Autodesk Inventor part; units mm, degrees
ref_plane "YZ Plane" through (0, 0, 0) normal (1, 0, 0) x (0, 1, 0)
ref_plane "XZ Plane" through (0, 0, 0) normal (0, 1, 0) x (-1, 0, 0)
ref_plane "XY Plane" through (0, 0, 0) normal (0, 0, 1) x (1, 0, 0)
sketch "Sketch1" plane through (0, 0, 0) normal (0, 0, 1) x (1, 0, 0)
  line L0 (262.89, 253.3796) -> (525.78, 101.6)
  line L1 (525.78, 101.6) -> (525.78, -201.9592) construction
  line L2 (525.78, -201.9592) -> (262.89, -353.7388) construction
  line L3 (262.89, -353.7388) -> (0, -201.9592) construction
  line L4 (0, -201.9592) -> (0, 101.6) construction
  line L5 (0, 101.6) -> (262.89, 253.3796)
  line L6 (0, 101.6) -> (0, 0)
  line L7 (0, 0) -> (525.78, 0)
  line L8 (525.78, 0) -> (525.78, 101.6)
  point P0 (262.89, -50.1796)
  dimension "d0" = 525.78
  dimension "d1" = 101.6
extrude "Extrusion1" add sketch "Sketch1" along normal blind 25.4
sketch "Sketch2" plane through (0, 0, 25.4) normal (0, 0, 1) x (1, 0, 0)
  circle A0 centre (262.89, 121.3796) radius 60
  line L0 (0, 0) -> (525.78, 0)
  point P0 (262.89, 0)
  dimension "d4" = 121.3796
  dimension "d5" = 120
extrude "Extrusion2" cut sketch "Sketch2" against normal through all
sketch "Sketch3" plane through (0, 0, 25.4) normal (0, 0, 1) x (1, 0, 0)
  circle A0 centre (262.89, 121.3796) radius 60
  line L0 (0, 101.6) -> (0, 0)
  line L1 (0, 0) -> (525.78, 0)
  line L2 (525.78, 0) -> (525.78, 101.6)
  line L3 (525.78, 101.6) -> (262.89, 253.3796)
  line L4 (262.89, 253.3796) -> (0, 101.6)
  line L5 (25.4, 86.9353) -> (25.4, 25.4)
  line L6 (25.4, 25.4) -> (500.38, 25.4)
  line L7 (500.38, 25.4) -> (500.38, 86.9353)
  line L8 (500.38, 86.9353) -> (262.89, 224.0502)
  line L9 (262.89, 224.0502) -> (25.4, 86.9353)
  dimension "d8" = 25.4
extrude "Extrusion3" cut sketch "Sketch3" against normal through all contours L4 L3 L2 L1 L0
sketch "Sketch4" plane through (0, 0, 25.4) normal (0, 0, 1) x (1, 0, 0)
  line L0 (134.346, 149.8353) -> (159.746, 105.8412)
  line L1 (159.746, 105.8412) -> (115.7519, 80.4412)
  line L2 (115.7519, 80.4412) -> (90.3519, 124.4353)
  line L3 (90.3519, 124.4353) -> (134.346, 149.8353)
  line L4 (134.346, 149.8353) -> (115.7519, 80.4412) construction
  line L5 (159.746, 105.8412) -> (90.3519, 124.4353) construction
  line L6 (262.89, 224.0502) -> (25.4, 86.9353)
  line L7 (500.38, 86.9353) -> (262.89, 224.0502)
  line L8 (262.89, 224.0502) -> (262.89, 25.4)
  line L9 (25.4, 25.4) -> (500.38, 25.4)
  line L10 (391.434, 149.8353) -> (366.034, 105.8412)
  line L11 (366.034, 105.8412) -> (410.0281, 80.4412)
  line L12 (410.0281, 80.4412) -> (435.4281, 124.4353)
  line L13 (435.4281, 124.4353) -> (391.434, 149.8353)
  line L14 (391.434, 149.8353) -> (410.0281, 80.4412) construction
  line L15 (366.034, 105.8412) -> (435.4281, 124.4353) construction
  point P0 (0, 0)
  point P1 (125.049, 115.1383)
  point P2 (400.731, 115.1383)
  point P3 (381.635, 155.4928)
  dimension "d11" = 50.8
  dimension "d12" = 50.8
  dimension "d15" = 75
extrude "Extrusion4" cut sketch "Sketch4" against normal through all
sketch "Sketch5" plane through (0, 0, 0) normal (0, 0, -1) x (-1, 0, 0)
  line L0 (-25.4, 86.9353) -> (-25.4, 25.4)
  line L1 (-25.4, 43.4677) -> (-12.7, 43.4677)
  line L2 (-12.7, 43.4677) -> (-12.7, 68.8677)
  line L3 (-12.7, 68.8677) -> (-25.4, 68.8677)
  line L4 (-25.4, 68.8677) -> (-25.4, 43.4677)
  line L5 (-25.4, 25.4) -> (-500.38, 25.4)
  line L6 (-94.99, 25.4) -> (-120.39, 25.4)
  line L7 (-120.39, 25.4) -> (-120.39, 12.7)
  line L8 (-120.39, 12.7) -> (-94.99, 12.7)
  line L9 (-94.99, 12.7) -> (-94.99, 25.4)
  line L10 (-405.39, 25.4) -> (-430.79, 25.4)
  line L11 (-430.79, 25.4) -> (-430.79, 12.7)
  line L12 (-430.79, 12.7) -> (-405.39, 12.7)
  line L13 (-405.39, 12.7) -> (-405.39, 25.4)
  line L14 (-500.38, 25.4) -> (-500.38, 86.9353)
  line L15 (-500.38, 43.4677) -> (-513.08, 43.4677)
  line L16 (-513.08, 43.4677) -> (-513.08, 68.8677)
  line L17 (-513.08, 68.8677) -> (-500.38, 68.8677)
  line L18 (-500.38, 68.8677) -> (-500.38, 43.4677)
  line L19 (-262.89, 224.0502) -> (-134.346, 149.8353)
  line L20 (-198.618, 186.9428) -> (-220.615, 199.6428)
  line L21 (-220.615, 199.6428) -> (-214.265, 210.6413)
  line L22 (-214.265, 210.6413) -> (-192.268, 197.9413)
  line L23 (-192.268, 197.9413) -> (-198.618, 186.9428)
  line L24 (-391.434, 149.8353) -> (-262.89, 224.0502)
  line L25 (-305.165, 199.6428) -> (-327.162, 186.9428)
  line L26 (-327.162, 186.9428) -> (-333.512, 197.9413)
  line L27 (-333.512, 197.9413) -> (-311.515, 210.6413)
  line L28 (-311.515, 210.6413) -> (-305.165, 199.6428)
  line L29 (-262.89, 224.0502) -> (-391.434, 149.8353)
  line L30 (-120.39, 19.05) -> (-405.39, 19.05) construction
  line L31 (-250.19, 25.4) -> (-275.59, 25.4)
  line L32 (-275.59, 25.4) -> (-275.59, 12.7)
  line L33 (-275.59, 12.7) -> (-250.19, 12.7)
  line L34 (-250.19, 12.7) -> (-250.19, 25.4)
  line L35 (-500.38, 25.4) -> (-25.4, 25.4)
  line L36 (-305.165, 199.6428) -> (-311.515, 210.6413)
  line L37 (-311.515, 210.6413) -> (-333.512, 197.9413)
  line L38 (-333.512, 197.9413) -> (-327.162, 186.9428)
  line L39 (-327.162, 186.9428) -> (-305.165, 199.6428)
  point P0 (0, 0)
  point P1 (-25.4, 56.1677)
  point P2 (-262.89, 25.4)
  point P3 (-262.89, 19.05)
  point P4 (-262.89, 25.4)
  dimension "d16" = 12.7
  dimension "d17" = 12.7
  dimension "d18" = 12.7
  dimension "d19" = 12.7
  dimension "d20" = 12.7
  dimension "d21" = 12.7
  dimension "d22" = 25.4
  dimension "d23" = 25.4
  dimension "d24" = 25.4
  dimension "d25" = 25.4
  dimension "d26" = 25.4
  dimension "d27" = 25.4
  dimension "d28" = 285
  dimension "d29" = 25.4
  dimension "d30" = 12.7
extrude "Extrusion5" add sketch "Sketch5" against normal blind 25.4
sketch "Sketch6" plane through (0, 0, 0) normal (0, 0, -1) x (-1, 0, 0)
  line L0 (-275.59, 25.4) -> (-405.39, 25.4)
  line L1 (-324.58, 25.4) -> (-375.38, 25.4)
  line L2 (-375.38, 25.4) -> (-375.38, 76.2)
  line L3 (-375.38, 76.2) -> (-324.58, 76.2)
  line L4 (-324.58, 76.2) -> (-324.58, 25.4)
  line L5 (-500.38, 43.4677) -> (-500.38, 25.4)
  point P0 (0, 0)
  dimension "d33" = 50.8
  dimension "d34" = 50.8
  dimension "d35" = 125
extrude "Extrusion6" cut sketch "Sketch6" against normal through all
sketch "Sketch8" plane through (500.38, 86.9353, 25.4) normal (0.5, 0.866, 0) x (0.866, -0.5, 0)
  circle A0 centre (-248.8298, 12.7) radius 2
  circle A1 centre (-25.4, 12.7) radius 2
  line L0 (0, 0) -> (0, 25.4)
  line L1 (-274.2298, 0) -> (-274.2298, 25.4)
  point P0 (-389.8741, 25.4)
  point P1 (0, 12.7)
  dimension "d44" = 4
  dimension "d45" = 4
  dimension "d46" = 25.4
  dimension "d47" = 25.4
extrude "Extrusion8" cut sketch "Sketch8" against normal blind 38.1
sketch "Sketch9" plane through (262.89, 224.0502, 25.4) normal (-0.5, 0.866, 0) x (0.866, 0.5, 0)
  line L0 (0, 0) -> (0, 25.4)
  line L1 (-274.2298, 0) -> (-274.2298, 25.4)
  circle A0 centre (-25.4, 12.7) radius 2
  circle A1 centre (-248.8298, 12.7) radius 2
  point P0 (-339.6945, 25.4)
  point P1 (-274.2298, 12.7)
  dimension "d50" = 4
  dimension "d51" = 4
  dimension "d52" = 25.4
  dimension "d53" = 25.4
extrude "Extrusion9" cut sketch "Sketch9" against normal blind 38.1
sketch "Sketch10" plane through (500.38, 25.4, 25.4) normal (1, 0, 0) x (0, 0, -1)
  line L0 (0, 0) -> (25.4, 0)
  line L1 (0, 61.5353) -> (25.4, 61.5353)
  circle A0 centre (12.7, 8) radius 2
  circle A1 centre (12.7, 53.5353) radius 2
  point P0 (25.4, -25.4)
  point P1 (12.7, 0)
  point P2 (12.7, 61.5353)
  dimension "d56" = 4
  dimension "d57" = 4
  dimension "d58" = 8
  dimension "d59" = 8
extrude "Extrusion10" cut sketch "Sketch10" against normal blind 38.1
sketch "Sketch11" plane through (25.4, 86.9353, 0) normal (-1, 0, 0) x (0, 0, 1)
  circle A0 centre (12.7, -8) radius 2
  circle A1 centre (12.7, -53.5353) radius 2
  point P0 (0, -86.9353)
extrude "Extrusion11" cut sketch "Sketch11" against normal blind 38.1
sketch "Sketch12" plane through (120.39, 25.4, 25.4) normal (0, -1, 0) x (1, 0, 0)
  circle A0 centre (-60.195, -12.7) radius 2
  circle A1 centre (64.9, -12.7) radius 2
  circle A2 centre (345.195, -12.7) radius 2
  line L0 (310.4, 0) -> (379.99, 0)
  line L1 (0, 0) -> (129.8, 0)
  line L2 (-94.99, 0) -> (-25.4, 0)
  line L3 (379.99, 0) -> (379.99, -25.4)
  point P0 (-120.39, -25.4)
  point P1 (345.195, 0)
  point P2 (64.9, 0)
  point P3 (-60.195, 0)
  point P4 (379.99, -12.7)
  dimension "d64" = 4
  dimension "d65" = 4
  dimension "d66" = 4
extrude "Extrusion12" cut sketch "Sketch12" against normal blind 38.1
properties part number "HB04" material "Polyethylene, High Density"
Here's how the part is built. I have some questions about the finished solid (model axes, mm). A direction names the side the tool comes from. Round coordinates to 2 decimals unless told otherwise and drop trailing zeros. Order: outer loops, then holes, each group sorted by start corner. A loop starts at its lowest first (then second) coordinate and runs counter-clockwise, first axis right, second up. Notation, with made-up numbers: (59, 27.5) -> (92, 27.5) arc R35 ccw to (92, 60.5) -> close; hole circle Ø8 at (-23.5, 55). An arc over 180 degrees is marked (long way). Return JSON: item names as keys, results as strings.
Q1. If we section it at D-D on x = 418: List the corners of the cut face in (y, z) for me, plus the area to 3 significant figures.
Filled sheet:
{"outline": "(12.7, 0) -> (94.25, 0) -> (94.25, 25.4) -> (12.7, 25.4) -> close", "area": "2,070 mm^2"}
Q2. If we section it at B-B on x = 299: List the corners of the cut face in (y, z) for me, plus the area to 3 significant figures.
Filled sheet:
{"outline": "(25.4, 0) -> (73.46, 0) -> (73.46, 25.4) -> (25.4, 25.4) -> close; (169.3, 0) -> (203.2, 0) -> (203.2, 25.4) -> (169.3, 25.4) -> close", "area": "2,080 mm^2"}
Q3. Which directions (+Z, -Z, +X, -X, +Y, -Y) give clear straight access to the entire face, cutting with the end or side of a thin tool? Please do faces 4 (the flat face through (500.38, 76, 13)), 5 (the flat face through (103.23, 102.13, 12.88)), 6 (the flat face through (146.868, 128.146, 12.878)).
Filled sheet:
{"face 4": "+Z, -Z, +X, +Y", "face 5": "+Z, -Z, +Y", "face 6": "+Z, -Z"}
Q4. I need wall thicknesses on line 1 along Z through (x, y) = (49, 33); line 2 along Y through (x, z) = (487, 12.7); line 3 along X through (y, z) = (87.5, 3.5). Which ranges of each line are inside material? Lowest first, please. Write a range as from..to.
Filled sheet:
{"line 1": "z = 0..10.74, 14.66..25.4", "line 2": "y = 25.4..31.4, 35.4..76.94, 80.94..94.66", "line 3": "x = 26.38..111.68, 127.98..213.37, 312.41..397.8, 414.1..499.4"}
Q5. If we mould it in two halves opening along X, with no side actions, what happens to faces 1 (the flat face through (19, 68.868, 13)), 2 (the flat face through (203.42, 204.38, 12.52)), 3 (the flat face through (324.58, 51, 13))? For each: released by +X, released by -X, zero draft, split by the parting line, or undercut.
Filled sheet:
{"face 1": "zero draft", "face 2": "released by -X", "face 3": "undercut"}
Q6. For pin 1 Ø3.5 at (y, z) = (78.94, 12.7) entering from +X; pin 2 Ø3 at (y, z) = (34, 12) entering from +X; pin 3 Ø10 at (y, z) = (18, 8.5) entering from +X, each with a flat end and sliding along its axis, tell me the tip position at first contact or that it passes through.
Filled sheet:
{"pin 1": "stops at x = 462.28", "pin 2": "stops at x = 500.38", "pin 3": "stops at x = 430.79"}
Q7. If we section it at A-A on y = 175.5: List the corners of the cut face in (x, z) for me.
Filled sheet:
{"outline": "(178.8, 0) -> (236.99, 0) -> (236.99, 25.4) -> (178.8, 25.4) -> close; (288.79, 0) -> (346.98, 0) -> (346.98, 25.4) -> (288.79, 25.4) -> close"}
Q8. If we section it at C-C on y = 94: Give the number of separate pieces and of enclosed holes in the cut face, plus the area to 3 significant figures.
Filled sheet:
{"separate pieces": "4", "enclosed holes": "2", "area": "7,110 mm^2"}
